from build123d import *

# Parameters (mm, degrees)
BOX001_W             = 21
BOX001_H             = 21
BOX001_DEPTH         = 24
FILLET_R             = 1
CONE_ROLL_ANGLE      = 0.050765
CONE_PITCH_ANGLE     = -7.966932
CONE_PLACEMENT_ANGLE = -0.72899
BOX_W                = 30
BOX_H                = 25
BOX_DEPTH            = 25
FILLET001_R          = 1


with BuildPart() as fillet_body:
    # Box001 → Box001 (new body)
    with BuildSketch(Plane(origin=(2, 2, 2), x_dir=(1, 0, 0), z_dir=(0, 0, 1))):
        with Locations((10.5, 10.5)):
            Rectangle(BOX001_W, BOX001_H)
    extrude(amount=BOX001_DEPTH)

    # Fillet
    fillet_edges = [fillet_body.edges().sort_by_distance(p)[0] for p in [
        (2, 2, 14),
        (2, 23, 14),
        (2, 12.5, 2),
        (23, 2, 14),
        (23, 23, 14),
        (23, 12.5, 2),
        (12.5, 2, 2),
        (12.5, 23, 2),
    ]]
    fillet(fillet_edges, radius=FILLET_R)


with BuildPart() as cone:
    # Cone → Cone (revolve)
    with BuildSketch(Plane.XZ):
        Polygon((0, 0), (5, 0), (1, 23), (0, 23), align=None)
    revolve(axis=Axis((0, 0, 0), (0, 0, 1)))


with BuildPart() as cone_1:
    # Cone roll: moved
    add(cone.part.rotate(Axis((0, 0, 0), (1, 0, 0)), CONE_ROLL_ANGLE))


with BuildPart() as cone_2:
    # Cone pitch: moved
    add(cone_1.part.rotate(Axis((0, 0, 0), (0, 1, 0)), CONE_PITCH_ANGLE))


with BuildPart() as cone_3:
    # Cone placement: moved
    add(cone_2.part.moved(Location((29, 12.5, -1))).rotate(Axis((29, 12.5, -1), (0, 0, 1)), CONE_PLACEMENT_ANGLE))


with BuildPart() as fillet001:
    # Box → Box (new body)
    with BuildSketch(Plane.XY):
        with Locations((15, 12.5)):
            Rectangle(BOX_W, BOX_H)
    extrude(amount=BOX_DEPTH)

    # Cut: cut Cone
    add(cone_3.part, mode=Mode.SUBTRACT)

    # Cut001: cut Fillet body
    add(fillet_body.part, mode=Mode.SUBTRACT)

    # Fillet001
    fillet001_edges = [fillet001.edges().sort_by_distance(p)[0] for p in [
        (0, 0, 12.5),
        (0, 12.5, 25),
        (0, 25, 12.5),
        (0, 12.5, 0),
        (15, 0, 0),
        (30, 0, 12.5),
        (15, 0, 25),
        (15, 25, 25),
        (30, 12.5, 25),
        (15, 25, 0),
        (30, 25, 12.5),
        (30, 21.109354, 0),
        (24.104388, 12.500455, 0),
        (30, 3.890653, 0),
    ]]
    fillet(fillet001_edges, radius=FILLET001_R)


solid = fillet001.part
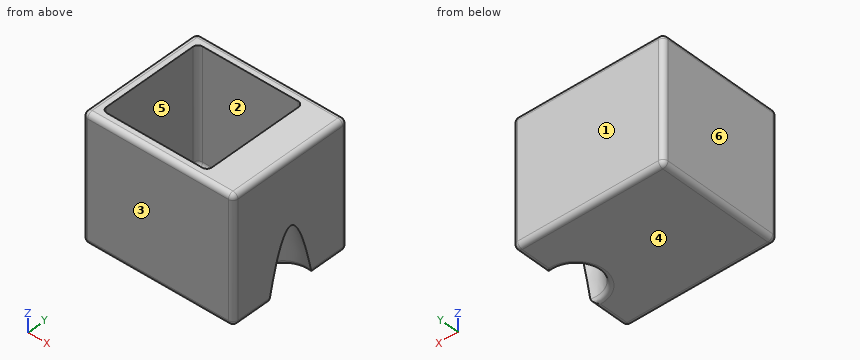
Work out the finished part from the listing and answer in its coordinate system (mm). Face numbers are marked on the shaded views. A direction names the side the tool comes from. Give positions to 0.01 mm unless a question says otherwise; leave off trailing zeros. Order: outer loops, then holes, each group sorted by start corner. A loop starts at its lowest first (then second) coordinate and runs counter-clockwise, first axis right, second up. Notation, with made-up numbers: (58, 71) -> (107, 71) arc R33 cw to (107, 108) -> close; hole circle Ø8 at (-10, 61). An arc over 180 degrees is marked (long way). Answer as a JSON object with one key per item and string values. Group by question number.
1. Consider line 1 along X through (y, z) = (6.5, 20.75); line 2 along Y through (x, z) = (19.5, 14.5); line 3 along X through (y, z) = (12, 18.25) (3 decimals). Determine where each line is inside the solid, lowest interval first. Write a range as [from, to].
2. Section C-C on y = 22.5 is taken. Determine the outline of the cut face in (x, z).
3. A tool of negligible diameter and unlimited length cuts with its end or side. For the marked faces 5 and 6, from which of +Z, -Z, +X, -X, +Y, -Y can it reach the whole face along a straight path? Write none if from no direction.
4. Section A-A on z = 22.75 is taken. Determine the outline of the cut face in (x, y), plus the area to 3 significant figures.
5. Section B-B on x = 17 is taken. Determine the outline of the cut face in (y, z), plus the area to 3 significant figures.
6. The mould has two halves that part along Y. Classify the marked faces 1, 2, 3 and 4: released by +Y, released by -Y, zero draft, split by the parting line, or undercut.
7. Section D-D on z = 15 is taken. Count the separate pieces of the cut face and the enclosed holes in it, plus the area to 3 significant figures.
8. Flat-ended cylindrical pins translate along their axes: pin 1 Ø5.5 at (x, y) = (8.5, 13.5) entering from +Z; pin 2 Ø3 at (x, y) = (8, 4) entering from +Z. Find the tip coordinate at first contact, or state that the pin passes through.
Result sheet:
{
 "1": {"line 1": "x = [0, 2], [23, 30]", "line 2": "y = [0, 2], [23, 25]", "line 3": "x = [0, 2], [23, 24.795], [27.897, 30]"},
 "2": {"outline": "(0, 1) arc R1 ccw to (1, 0) -> (29, 0) arc R1 ccw to (30, 1) -> (30, 24) arc R1 ccw to (29, 25) -> (22.87, 25) -> (22.87, 3) arc R0.87 cw to (22, 2.13) -> (3, 2.13) arc R0.87 cw to (2.13, 3) -> (2.13, 25) -> (1, 25) arc R1 ccw to (0, 24) -> close"},
 "3": {"face 5": "+Z", "face 6": "+Z, -Z, -X, +Y, -Y"},
 "4": {"outline": "(0, 1) arc R1 ccw to (1, 0) -> (29, 0) arc R1 ccw to (30, 1) -> (30, 24) arc R1 ccw to (29, 25) -> (1, 25) arc R1 ccw to (0, 24) -> close; hole (2, 3) arc R1 ccw to (3, 2) -> (22, 2) arc R1 ccw to (23, 3) -> (23, 22) arc R1 ccw to (22, 23) -> (3, 23) arc R1 ccw to (2, 22) -> close", "area": "309 mm^2"},
 "5": {"outline": "(0, 1) arc R1 ccw to (1, 0) -> (24, 0) arc R1 ccw to (25, 1) -> (25, 24) arc R1 ccw to (24, 25) -> (23, 25) -> (23, 3) arc R1 cw to (22, 2) -> (3, 2) arc R1 cw to (2, 3) -> (2, 25) -> (1, 25) arc R1 ccw to (0, 24) -> close", "area": "142 mm^2"},
 "6": {"face 1": "released by +Y", "face 2": "undercut", "face 3": "released by -Y", "face 4": "zero draft"},
 "7": {"separate pieces": "1", "enclosed holes": "2", "area": "294 mm^2"},
 "8": {"pin 1": "stops at z = 2", "pin 2": "stops at z = 2.13"}
}
